Input: part model. Units: mm. Frame: model coordinates. Face numbers are marked on the shaded views. A direction names the side the tool comes from. Coordinates: 2 decimals unless noted, no trailing zeros. Order: outer loops, then holes, each group sorted by start corner. A loop starts at its lowest first (then second) coordinate and runs counter-clockwise, first axis right, second up. Notation, with made-up numbers: (88, 71) -> (140, 71) arc R31 cw to (140, 97) -> close; hole circle Ø9 at (34.25, 13). An arc over 180 degrees is marked (long way). Write each question's results on one line, items separated by ' | '.
```python
from build123d import *

# Parameters (mm, degrees)
EXTRUDE_1_DEPTH        = 1
CHAMFER_1_SIZE         = 1
CHAMFER_1_SIZE2        = 0.577350269
CHAMFER_1_PART_2_SIZE  = 1
CHAMFER_1_PART_2_SIZE2 = 0.577350269
CHAMFER_1_PART_3_SIZE  = 1
CHAMFER_1_PART_3_SIZE2 = 0.577350269
CHAMFER_1_PART_4_SIZE  = 1
CHAMFER_1_PART_4_SIZE2 = 0.577350269


with BuildPart() as part:
    # Эскиз1 → Бобышка-Вытянуть1 (new body, symmetric)
    with BuildSketch(Plane.XY):
        Polygon((1, 0), (-1, 0), (-1, 5), (-2.75, 5), (-2.75, 6.6), (-2, 6.6), (-2, 18.6), (2, 18.6), (2, 6.6), (2.75, 6.6), (2.75, 5), (1, 5), align=None)
    extrude(amount=EXTRUDE_1_DEPTH, both=True)

    # Фаска1
    chamfer_1_edges = [part.edges().sort_by_distance(p)[0] for p in [
        (0, 18.6, -1),
    ]]
    chamfer_1_side = [part.faces().sort_by_distance(p)[0] for p in [
        (0, 10.192215569, -1),
    ]]
    chamfer(chamfer_1_edges, length=CHAMFER_1_SIZE, length2=CHAMFER_1_SIZE2, reference=chamfer_1_side[0])

    # Фаска1 part 2
    chamfer_1_part_2_edges = [part.edges().sort_by_distance(p)[0] for p in [
        (-2, 18.6, 0),
    ]]
    chamfer_1_part_2_side = [part.faces().sort_by_distance(p)[0] for p in [
        (-2, 12.6, 0),
    ]]
    chamfer(chamfer_1_part_2_edges, length=CHAMFER_1_PART_2_SIZE, length2=CHAMFER_1_PART_2_SIZE2, reference=chamfer_1_part_2_side[0])

    # Фаска1 part 3
    chamfer_1_part_3_edges = [part.edges().sort_by_distance(p)[0] for p in [
        (2, 18.6, 0),
    ]]
    chamfer_1_part_3_side = [part.faces().sort_by_distance(p)[0] for p in [
        (2, 12.6, 0),
    ]]
    chamfer(chamfer_1_part_3_edges, length=CHAMFER_1_PART_3_SIZE, length2=CHAMFER_1_PART_3_SIZE2, reference=chamfer_1_part_3_side[0])

    # Фаска1 part 4
    chamfer_1_part_4_edges = [part.edges().sort_by_distance(p)[0] for p in [
        (0, 18.6, 1),
    ]]
    chamfer_1_part_4_side = [part.faces().sort_by_distance(p)[0] for p in [
        (0, 10.192215569, 1),
    ]]
    chamfer(chamfer_1_part_4_edges, length=CHAMFER_1_PART_4_SIZE, length2=CHAMFER_1_PART_4_SIZE2, reference=chamfer_1_part_4_side[0])


solid = part.part
```
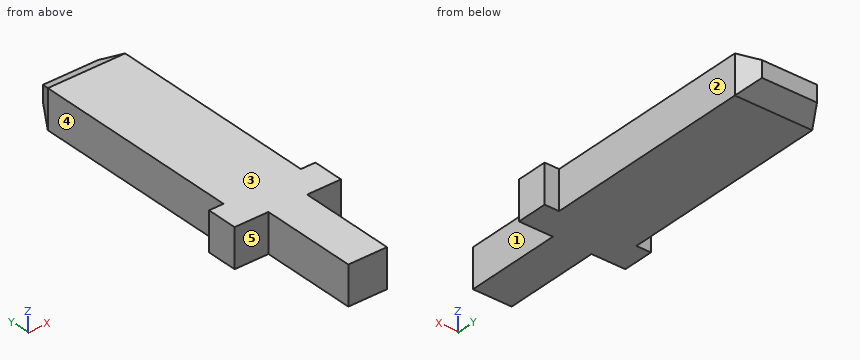
(1) Cut plane B-B, the plane x = 0. Return loops of the section in (y, z).
Return value:
outline: (0, -1) -> (17.6, -1) -> (18.6, -0.42) -> (18.6, 0.42) -> (17.6, 1) -> (0, 1) -> close
(2) Cut plane D-D, the plane z = -0.6. Return loops of the section in (x, y).
Return value:
outline: (-2.75, 5) -> (-1, 5) -> (-1, 0) -> (1, 0) -> (1, 5) -> (2.75, 5) -> (2.75, 6.6) -> (2, 6.6) -> (2, 17.6) -> (1.6, 18.29) -> (-1.6, 18.29) -> (-2, 17.6) -> (-2, 6.6) -> (-2.75, 6.6) -> close
(3) Cut plane C-C, the plane y = 14. Return loops of the section in (x, z), plus the area to 3 significant figures.
Return value:
outline: (-2, -1) -> (2, -1) -> (2, 1) -> (-2, 1) -> close | area: 8.00 mm2
(4) Line query: line 1 along X through (y, z) = (1, -0.65); line 2 along Y through (x, z) = (-2.4, -0.75); line 3 along Y through (x, z) = (-1.05, -0.35). Output: solid intervals per line, ascending. Write a range as from..to.
Return value:
line 1: -1..1 | line 2: 5..6.6 | line 3: 5..18.6
(5) Pin query (flat end, axial travel): P1, Ø1, axis at y = 12, z = -0.5, coming from the -X side; P2, Ø0.6, axis at x = 2.5, z = -0.5, coming from the +Y side; P3, Ø1, axis at y = 2.5, z = 0, coming from the -X side. Return the tip coordinate at first contact, or that it passes through.
Return value:
P1: x = -2 | P2: y = 6.6 | P3: x = -1
(6) Cut plane A-A, the plane z = 0.1. Return loops of the section in (x, y).
Return value:
outline: (-2.75, 5) -> (-1, 5) -> (-1, 0) -> (1, 0) -> (1, 5) -> (2.75, 5) -> (2.75, 6.6) -> (2, 6.6) -> (2, 17.6) -> (1.42, 18.6) -> (-1.42, 18.6) -> (-2, 17.6) -> (-2, 6.6) -> (-2.75, 6.6) -> close
(7) Reachability of the marked faces 1, 2, 3, 4 and 5 from +Z, -Z, +X, -X, +Y, -Y: full face, straight path, thin tool, end or side. Return the list, or none.
Return value:
face 1: +Z, -Z, +X, -Y | face 2: +Z, -Z, +X, +Y | face 3: +Z, +X, -X, +Y, -Y | face 4: +Z, -Z, -X, +Y | face 5: +Z, -Z, -X, -Y
